```python
from build123d import *

# Parameters (mm, degrees)
F1_DEPTH = 10.5
F2_R     = 1.75
F3_DEPTH = 50
F2_R_2   = 3.5
F4_DEPTH = 5
F2_R_3   = 2.05
F5_DEPTH = 20
F8_DEPTH = 4


with BuildPart() as f1:
    # F0 (on Front) → F1 (new body)
    with BuildSketch(Plane.XZ):
        Polygon((9.366447, 24.13893), (1.366447, 24.13893), (1.366447, -28.36107), (12.366447, -28.36107), (12.366447, -3.36107), (8.366447, -3.36107), (8.366447, 11.63893), (12.366447, 11.63893), (12.366447, 24.13893), align=None)
    extrude(amount=F1_DEPTH)

    # F2 (on Right) → F3 (cut)
    with BuildSketch(Plane.YZ):
        with Locations((-5.25, -9.61107)):
            Circle(F2_R)
        with Locations((-5.25, 17.88893)):
            Circle(F2_R)
    extrude(amount=F3_DEPTH, mode=Mode.SUBTRACT)

    # F2 (on Right) → F4 (cut)
    with BuildSketch(Plane.YZ):
        with Locations((-5.25, -9.61107)):
            Circle(F2_R_2)
        with Locations((-5.25, -9.61107)):
            Circle(F2_R, mode=Mode.SUBTRACT)
        with Locations((-5.25, 17.88893)):
            Circle(F2_R_2)
        with Locations((-5.25, 17.88893)):
            Circle(F2_R, mode=Mode.SUBTRACT)
    extrude(amount=F4_DEPTH, mode=Mode.SUBTRACT)

    # F2 (on Right) → F5 (cut)
    with BuildSketch(Plane.YZ):
        with Locations((-5.256939, -20.86107)):
            Circle(F2_R_3)
        with Locations((-5.25, 9.13893)):
            Circle(F2_R_3)
    extrude(amount=F5_DEPTH, mode=Mode.SUBTRACT)

    # F7 (on offset) → F8 (cut)
    with BuildSketch(Plane.YZ.offset(7.5)):
        Polygon((-6.44787, -16.527179), (-9.611129, -19.727772), (-8.420963, -24.06753), (-4.067539, -25.206696), (-0.90428, -22.006103), (-2.094446, -17.666345), align=None)
        Polygon((-6.461621, 13.450113), (-9.632396, 10.256967), (-8.452437, 5.914422), (-4.101703, 4.765023), (-0.930928, 7.95817), (-2.110887, 12.300715), align=None)
    extrude(amount=-F8_DEPTH, mode=Mode.SUBTRACT)


solid = f1.part
```
Source: CAD feature listing. Evaluate the final solid. Frame: model axes, mm. A direction names the side the tool comes from. Give positions to 0.01 mm unless a question says otherwise; leave off trailing zeros. Write each loop counter-clockwise with the first axis right and the second up, starting at its lowest first coordinate (ties: lowest second). Pieces come first, ordered by that corner, then holes.
1. Access query for faces 4 (the face through (5.53, -9.05, 8.12)), 5 (the face through (8.632, -6.639, -10.676)), 6 (the face through (10, -5, -3.361)). Directions: +Z, -Z, +X, -X, +Y, -Y. A direction counts if a zero-diameter tool reaches every point of the face in a straight line with its end or side. Return the directions, or none.
2. First-contact query: pin 1 (3 mm diameter, centred on y = -6.5, z = 6, fed in from +X); pin 2 (5.5 mm diameter, centred on y = -5.25, z = -9.61, fed in from -X); pin 3 (3.5 mm diameter, centred on y = -5.26, z = -20.86, fed in from +X). Flat tips, straight axial feed; report the tip coordinate or a pass-through.
3. Section query B-B (y = -5.25). Count the separate pieces of the cut face and the enclosed holes in it, then the cut area to 3 significant figures.
4. Material intervals for line 1 along Z through (x, y) = (7.75, -5.25); line 2 along Z through (x, y) = (10, -8.5); line 3 along Z through (x, y) = (4.75, -2.25), sorted ascending.
5. Section query C-C (z = 0). Return the cut outline in (x, y), then the cut area to 3 significant figures.
6. Section query A-A (x = 2.5). Return the cut outline in (y, z).
7. Pull-direction query (Z, two-part tool) for faces 1 (the face through (7, 0, -2)), 2 (the face through (7, -5, -28.361)), 3 (the face through (7.5, -6, 7)); classes: +Z half, -Z half, draft (parallel to the pull), parting line (faces both ways), or undercut.
Output values:
1. face 4: none
1. face 5: +X, -X
1. face 6: +X, +Y, -Y
2. pin 1: stops at x = 8.37
2. pin 2: stops at x = 5
2. pin 3: passes through
3. separate pieces: 5
3. enclosed holes: 0
3. area: 310 mm2
4. line 1: z = -28.36 to -22.91, -18.81 to -11.36, -7.86 to 7.09, 11.19 to 16.14, 19.64 to 24.14
4. line 2: z = -28.36 to -3.36, 11.64 to 24.14
4. line 3: z = -28.36 to -23.37, -17.63 to -11.41, -7.81 to 6.63, 12.34 to 16.09, 19.69 to 24.14
5. outline: (1.37, -10.5) - (8.37, -10.5) - (8.37, 0) - (1.37, 0) - close
5. area: 73.5 mm2
6. outline: (-10.5, -28.36) - (0, -28.36) - (0, 24.14) - (-10.5, 24.14) - close; hole circle Ø7 at (-5.25, -9.61); hole circle Ø7 at (-5.25, 17.89); hole circle Ø4.1 at (-5.26, -20.86); hole circle Ø4.1 at (-5.25, 9.14)
7. face 1: draft
7. face 2: -Z half
7. face 3: undercut
